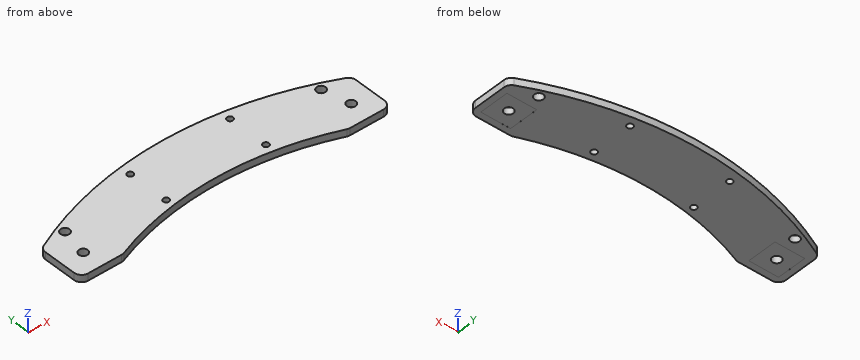
from build123d import *

# Parameters (mm, degrees)
SKETCH1_R           = 2
SKETCH1_R_2         = 3
BOSS_EXTRUDE1_DEPTH = 4.7625
SKETCH4_W           = 20
SKETCH4_H           = 20
CUT_EXTRUDE2_DEPTH  = 0.01


with BuildPart() as part:
    # Sketch1 → Boss-Extrude1 (new body)
    with BuildSketch(Plane.XY):
        with BuildLine():
            Line((-14.25, -9.25), (-14.25, 12.676812237))
            ThreePointArc((-14.25, 12.676812237), (-13.494277193, 15.319937491), (-11.455555556, 17.164074731))
            ThreePointArc((-11.455555556, 17.164074731), (90, 40.75), (191.455555556, 17.164074731))
            ThreePointArc((191.455555556, 17.164074731), (193.494277193, 15.319937491), (194.25, 12.676812237))
            Line((194.25, 12.676812237), (194.25, -9.25))
            ThreePointArc((194.25, -9.25), (192.785533906, -12.785533906), (189.25, -14.25))
            Line((189.25, -14.25), (166.727208071, -14.25))
            ThreePointArc((166.727208071, -14.25), (165.774029952, -14.158304338), (164.855812752, -13.886580589))
            ThreePointArc((164.855812752, -13.886580589), (90, 0.65019584), (15.144187248, -13.886580589))
            ThreePointArc((15.144187248, -13.886580589), (14.225970048, -14.158304338), (13.272791929, -14.25))
            Line((13.272791929, -14.25), (-9.25, -14.25))
            ThreePointArc((-9.25, -14.25), (-12.785533906, -12.785533906), (-14.25, -9.25))
        make_face()
        with Locations((59, 31.25)):
            Circle(SKETCH1_R, mode=Mode.SUBTRACT)
        with Locations((59, 3.75)):
            Circle(SKETCH1_R, mode=Mode.SUBTRACT)
        with Locations((126, 31.25)):
            Circle(SKETCH1_R, mode=Mode.SUBTRACT)
        with Locations((126, 3.75)):
            Circle(SKETCH1_R, mode=Mode.SUBTRACT)
        with Locations((180, 0)):
            Circle(SKETCH1_R_2, mode=Mode.SUBTRACT)
        Circle(SKETCH1_R_2, mode=Mode.SUBTRACT)
        with Locations((4, 18.5)):
            Circle(SKETCH1_R_2, mode=Mode.SUBTRACT)
        with Locations((176, 18.5)):
            Circle(SKETCH1_R_2, mode=Mode.SUBTRACT)
    extrude(amount=BOSS_EXTRUDE1_DEPTH)

    # Sketch4 → Cut-Extrude2 (cut)
    with BuildSketch(Plane.XY):
        Rectangle(SKETCH4_W, SKETCH4_H)
        with Locations((180, 0)):
            Rectangle(SKETCH4_W, SKETCH4_H)
    extrude(amount=CUT_EXTRUDE2_DEPTH, mode=Mode.SUBTRACT)


solid = part.part
Work out the finished part from the listing and answer in its coordinate system (mm). Round coordinates to 2 decimals unless told otherwise and drop trailing zeros. Loops run counter-clockwise (first coordinate to the right, second up) from the corner with the lowest first, then second, coordinate; pieces in that order, holes last. Notation, with made-up numbers: (17.25, 65) - (42.25, 65) arc R7 ccw to (42.25, 76) - close; hole circle Ø10 at (13.5, 64.5). An arc over 180 degrees is marked (long way). One line per item, written item: value.
Q1. Straight lines are drawn through the part: probe 1 along Y at (x, z) = (177.5, 3.4); probe 2 along Y at (x, z) = (126, 2.85); probe 3 along Y at (x, z) = (0, 0.6). For each, find the intervals that lie inside material, in ascending order.
Check values:
probe 1: -14.25 to -1.66, 1.66 to 15.9, 21.1 to 23.46
probe 2: -2.62 to 1.75, 5.75 to 29.25, 33.25 to 37.92
probe 3: -14.25 to -3, 3 to 22.41
Q2. Find section D-D on x = 126. Give the vertices of the cut face in (y, z).
Check values:
outline: (-2.62, 0) - (1.75, 0) - (1.75, 4.76) - (-2.62, 4.76) - close; (5.75, 0) - (29.25, 0) - (29.25, 4.76) - (5.75, 4.76) - close; (33.25, 0) - (37.92, 0) - (37.92, 4.76) - (33.25, 4.76) - close
Q3. Find section A-A on x = 59. Give the vertices of the cut face in (y, z), and give its area (3 significant figures).
Check values:
outline: (-1.77, 0) - (1.75, 0) - (1.75, 4.76) - (-1.77, 4.76) - close; (5.75, 0) - (29.25, 0) - (29.25, 4.76) - (5.75, 4.76) - close; (33.25, 0) - (38.65, 0) - (38.65, 4.76) - (33.25, 4.76) - close
area: 154 mm2
Q4. Find section B-B on z = 3.85. State how many separate pieces and enclosed holes the cut face has, and give its area (3 significant figures).
Check values:
separate pieces: 1
enclosed holes: 8
area: 8,080 mm2
Q5. This flat-tipped pin is pushed along its axis until it touches: pin 1 Ø6 at (x, y) = (-5, 3) entering from -Z. Where does it stop, or does it pass through?
Check values:
pin 1: z = 0.01
Q6. Find section C-C on y = 27.5. Give the vertices of the cut face in (x, z), and give its area (3 significant figures).
Check values:
outline: (13.06, 0) - (166.94, 0) - (166.94, 4.76) - (13.06, 4.76) - close
area: 733 mm2
